Autodesk Inventor part; units mm, degrees
ref_plane "YZ Plane" through (0, 0, 0) normal (1, 0, 0) x (0, 1, 0)
ref_plane "XZ Plane" through (0, 0, 0) normal (0, 1, 0) x (-1, 0, 0)
ref_plane "XY Plane" through (0, 0, 0) normal (0, 0, 1) x (1, 0, 0)
sketch "Sketch1" plane through (0, 0, 0) normal (1, 0, 0) x (0, 1, 0)
  line L0 (5, 0) -> (70, 0)
  line L1 (70, 0) -> (70, -20)
  line L2 (70, -20) -> (0, -20)
  line L3 (0, -5) -> (0, -5)
  circle A0 centre (60, -10) radius 1.75
  circle A1 centre (40, -10) radius 1.75
  line L4 (0, -20) -> (-45, -20)
  line L5 (-45, -20) -> (-45, -10)
  line L6 (-40, -5) -> (0, -5)
  arc A2 (5, 0) -> (0, -5) centre (5, -5) ccw
  arc A3 (-40, -5) -> (-45, -10) centre (-40, -10) ccw
  point P0 (0, 0)
  point P1 (-45, -5)
  dimension "d0" = 70
  dimension "d1" = 20
  dimension "d4" = 3.5
  dimension "d5" = 3.5
  dimension "d6" = 45
  dimension "d7" = 15
  dimension "d8" = 5
extrude "Extrusion1" add sketch "Sketch1" along normal blind 4
sketch "Sketch2" plane through (4, 0, 0) normal (1, 0, 0) x (0, 0, -1)
  arc A0 (5, -40) -> (10, -45) centre (10, -40) ccw
  line L0 (20, -52) -> (10, -52)
  line L1 (5, -47) -> (5, -40)
  arc A1 (5, -47) -> (10, -52) centre (10, -47) ccw
  line L2 (20, -52) -> (20, -49)
  line L3 (20, -49) -> (15, -49)
  line L4 (15, -49) -> (15, -39)
  line L5 (15, -39) -> (20, -39)
  line L6 (5, -40) -> (15, -40)
  point P0 (0, 0)
  point P1 (5, -52)
  dimension "d11" = 15
  dimension "d13" = 5
  dimension "d14" = 3
  dimension "d15" = 5
  dimension "d16" = 10
extrude "Extrusion2" add sketch "Sketch2" against normal blind 4
sketch "Sketch3" plane through (4, 0, 0) normal (1, 0, 0) x (0, 0, -1)
  line L0 (15, -45) -> (20, -45)
  line L1 (15, -45) -> (20, -45)
  line L2 (20, -45) -> (20, -44)
  line L3 (20, -44) -> (15, -44)
  line L4 (15, -44) -> (15, -45)
  point P0 (0, 0)
  dimension "d19" = 5
  dimension "d20" = 1
extrude "Extrusion3" cut sketch "Sketch3" against normal blind 4
properties part number "g_griper left jaw_arm"
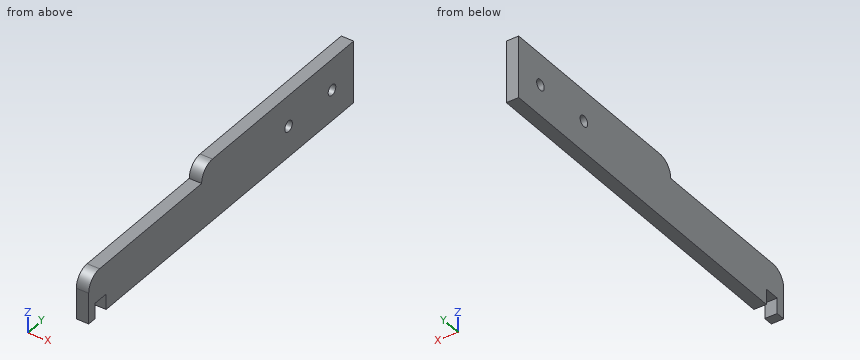
Can you work these out from the model? Positions are in its coordinate system, mm. Round coordinates to 2 decimals unless told otherwise and drop trailing zeros. Order: outer loops, then holes, each group sorted by start corner. A loop starts at its lowest first (then second) coordinate and runs counter-clockwise, first axis right, second up. Notation, with made-up numbers: (-6, 87.5) - (-1, 87.5) arc R20 cw to (-1, 121.5) - close; hole circle Ø9 at (23.5, -33). An arc over 180 degrees is marked (long way). Answer in a Markdown table with one row per item.
(1) Suppose I cut it at D-D, the plane y = -2.5. Please give me the cut outline in (x, z).
From the geometry:
| item | result |
|---|---|
| outline | (0, -20) - (4, -20) - (4, -5) - (0, -5) - close |
(2) Suppose I cut it at C-C, the plane y = 40. Please give me the cut outline in (x, z).
From the geometry:
| item | result |
|---|---|
| outline | (0, -20) - (4, -20) - (4, -11.75) - (0, -11.75) - close; (0, -8.25) - (4, -8.25) - (4, 0) - (0, 0) - close |
(3) Suppose I cut it at A-A, the plane x = 2.55. Please give me the cut outline in (y, z).
From the geometry:
| item | result |
|---|---|
| outline | (-52, -20) - (-49, -20) - (-49, -15) - (-44, -15) - (-44, -20) - (70, -20) - (70, 0) - (5, 0) arc R5 ccw to (0, -5) - (-47, -5) arc R5 ccw to (-52, -10) - close; hole circle Ø3.5 at (40, -10); hole circle Ø3.5 at (60, -10) |
(4) Please list where these lines run through material, in increasing order: L1, parallel to Z at x = 1.6, y = 60; L2, parallel to Y at x = 1.75, z = -11.5; L3, parallel to Y at x = 2.45, z = -18.5. Write a range as from..to.
From the geometry:
| item | result |
|---|---|
| L1 | z = -20..-11.75, -8.25..0 |
| L2 | y = -52..39.1, 40.9..59.1, 60.9..70 |
| L3 | y = -52..-49, -44..70 |
(5) Suppose I cut it at B-B, the plane z = -16. Please give me the cut outline in (x, y).
From the geometry:
| item | result |
|---|---|
| outline | (0, -52) - (4, -52) - (4, -49) - (0, -49) - close; (0, -44) - (4, -44) - (4, 70) - (0, 70) - close |
(6) For P1, Ø8, axis at y = -39.5, z = -13, coming from the -X side; P2, Ø3, axis at y = 40, z = -10, coming from the +X side, each with a flat end and sliding along its axis, tell me the tip position at first contact or that it passes through.
From the geometry:
| item | result |
|---|---|
| P1 | stops at x = 0 |
| P2 | passes through |
